```python
from build123d import *

# Parameters (mm, degrees)
F0_W     = 76.2
F0_H     = 76.2
F1_DEPTH = 76.2
F2_R     = 19.05
F3_DEPTH = 76.201
F4_R     = 19.05
F5_DEPTH = 76.2


with BuildPart() as f1:
    # F0 (on Front) → F1 (new body)
    with BuildSketch(Plane.XZ):
        with Locations((38.1, 38.1)):
            Rectangle(F0_W, F0_H)
    extrude(amount=F1_DEPTH)

    # F2 (on face) → F3 (cut, through all)
    with BuildSketch(Plane.YZ.offset(76.2)):
        with Locations((-38.1, 38.1)):
            Circle(F2_R)
    extrude(amount=-F3_DEPTH, mode=Mode.SUBTRACT)

    # F4 (on face) → F5 (cut)
    with BuildSketch(Plane.XZ.offset(76.2)):
        with Locations((38.1, 38.1)):
            Circle(F4_R)
    extrude(amount=-F5_DEPTH, mode=Mode.SUBTRACT)


solid = f1.part
```
Design review of the part built by this model. Coordinates are the model's own, in mm. Round coordinates to 2 decimals unless told otherwise and drop trailing zeros. Order: outer loops, then holes, each group sorted by start corner. A loop starts at its lowest first (then second) coordinate and runs counter-clockwise, first axis right, second up. Notation, with made-up numbers: (-40, 47.5) - (-5, 47.5) arc R23 cw to (-5, 63.5) - close; hole circle Ø8 at (-36.75, -31). An arc over 180 degrees is marked (long way). One line per question, with ' | ' between items.
Item 1: Take a section at B-B, the plane y = -10. Write out the cut boundary in (x, z), then the cut area to 3 significant figures.
Checks:
outline: (0, 0) - (76.2, 0) - (76.2, 76.2) - (0, 76.2) - close; hole circle Ø38.1 at (38.1, 38.1) | area: 4,670 mm²
Item 2: For P1, Ø23, axis at y = -38.1, z = 38.1, coming from the +X side, flat-tipped, find the tip position at first contact; note if it passes through.
Checks:
P1: through
Item 3: Wall thickness on line 1 (X direction, y = -13, z = 38); line 2 (Y direction, x = 17, z = 38.1): over which ranges is each line inside the solid? List them lowest first. Write a range as [from, to].
Checks:
line 1: [0, 19.05], [57.15, 76.2] | line 2: [-76.2, -57.15], [-19.05, 0]
Item 4: Take a section at A-A, the plane z = 38.1. Write out the cut boundary in (x, y), then the cut area to 3 significant figures.
Checks:
outline: (0, -76.2) - (19.05, -76.2) - (19.05, -57.15) - (0, -57.15) - close; (0, -19.05) - (19.05, -19.05) - (19.05, 0) - (0, 0) - close; (57.15, -76.2) - (76.2, -76.2) - (76.2, -57.15) - (57.15, -57.15) - close; (57.15, -19.05) - (76.2, -19.05) - (76.2, 0) - (57.15, 0) - close | area: 1,450 mm²
Item 5: Take a section at C-C, the plane y = -51.5. Write out the cut boundary in (x, z), then the cut area to 3 significant figures.
Checks:
outline: (0, 0) - (76.2, 0) - (76.2, 24.56) - (51.5, 24.56) arc R19.05 cw to (24.7, 24.56) - (0, 24.56) - close; (0, 51.64) - (24.7, 51.64) arc R19.05 cw to (51.5, 51.64) - (76.2, 51.64) - (76.2, 76.2) - (0, 76.2) - close | area: 3,540 mm²
Item 6: Take a section at D-D, the plane x = 30. Write out the cut boundary in (y, z).
Checks:
outline: (-76.2, 0) - (0, 0) - (0, 20.86) - (-30, 20.86) arc R19.05 cw to (-46.2, 20.86) - (-76.2, 20.86) - close; (-76.2, 55.34) - (-46.2, 55.34) arc R19.05 cw to (-30, 55.34) - (0, 55.34) - (0, 76.2) - (-76.2, 76.2) - close
Item 7: Draft analysis for pull direction X (two halves, no side actions). For faces 1 (the face through (76.2, -29, 21)), 2 (the face through (29, -76.2, 56)), 3 (the face through (0, -29, 21)), 4 (the face through (48.341, -61.65, 54.163)), state which applies: +X half, -X half, draft (parallel to the pull), parting line (faces both ways), or undercut.
Checks:
face 1: +X half | face 2: draft | face 3: -X half | face 4: undercut
